Autodesk Inventor part; units mm, degrees
ref_plane "YZ Plane" through (0, 0, 0) normal (1, 0, 0) x (0, 1, 0)
ref_plane "XZ Plane" through (0, 0, 0) normal (0, 1, 0) x (-1, 0, 0)
ref_plane "XY Plane" through (0, 0, 0) normal (0, 0, 1) x (1, 0, 0)
sketch "Sketch1" plane through (0, 0, 0) normal (0, 1, 0) x (-1, 0, 0)
  line L0 (0, 0) -> (0, 19.05)
  line L1 (0, 19.05) -> (0.7937, 19.05)
  line L2 (0.7937, 19.05) -> (0.7938, 0.7937)
  line L3 (0.7938, 0.7937) -> (19.05, 0.7937)
  line L4 (19.05, 0.7937) -> (19.05, 0)
  line L5 (19.05, 0) -> (0, 0)
  dimension "d0" = 19.05
  dimension "d1" = 0.7937
extrude "Extrusion1" add sketch "Sketch1" along normal blind 76.2
sketch "Sketch2" plane through (0, 0, 19.05) normal (1, 0, 0) x (0, 0, -1)
  circle A0 centre (9.1281, 69.85) radius 3.3782
  circle A1 centre (9.1281, 44.45) radius 3.3782
  line L0 (0, 76.2) -> (19.05, 76.2)
  line L1 (0, 0) -> (0, 76.2)
  line L2 (18.2563, 0) -> (18.2563, 76.2)
  line L3 (18.2563, 38.1) -> (0, 38.1) construction
  line L4 (9.1281, 38.1) -> (9.1281, 76.2) construction
  dimension "d5" = 6.7564
  dimension "d18" = 25.4
  dimension "d19" = 6.35
extrude "Extrusion2" cut sketch "Sketch2" against normal through all
properties part number "Shooter Main Gear Guide Bar" material "Aluminum 6061"
Geometry check sheet. Reference: the model listing, model coordinates, mm. A direction names the side the tool comes from. Coordinates: 2 decimals unless noted, no trailing zeros. Write each loop counter-clockwise with the first axis right and the second up, starting at its lowest first coordinate (ties: lowest second). Pieces come first, ordered by that corner, then holes. Notation, with made-up numbers: M 73,-13.5 L 118,-13.5 A29 ccw 118,21.5 Z; hole C 70.25,-15.75 d5. An arc over 180 degrees is marked long. Use one line per item in the form item = value. Start each with the question number.
1) Set-up check for faces 1 (the flat face through (-0.3, 76.2, 5.3)), 2 (the flat face through (-10, 38, 0.794)): record each of +Z, -Z, +X, -X, +Y, -Y from which the full face is reachable in a straight line by a thin tool's end or side.
2) Release check for a two-part mould opening along Y. For faces 3 (the flat face through (-10, 38, 0)), 4 (the cylindrical face through (-0.391, 66.853, 8.363)), 5 (the flat face through (-0.3, 0, 5.3)), 6 (the cylindrical face through (-0.39, 41.15, 10.65)) record: pulls with the +Y half, pulls with the -Y half, needs draft (parallel to the pull), parting line crosses it, or undercut.
3) Section check C-C on y = 34. Enter the section's corners in (x, z).
4) Section check A-A on z = 10.25. Enter the section's corners in (x, y).
5) Section check B-B on y = 69.85. Enter the section's corners in (x, z), and give its area (3 significant figures).
6) Thickness scan on probe 1 along Z at (x, y) = (-0.2, 44.45); probe 2 along X at (y, z) = (71.5, 3); probe 3 along Z at (x, y) = (-7, 13). Record the ranges inside material, lowest first. Write a range as from..to.
7) Go/stop test with flat-tipped pins: pin 1 Ø4 at (x, y) = (-13.5, 61) entering from +Z; pin 2 Ø9 at (y, z) = (39.5, 6.5) entering from -X. Record where each tip stops, or that it passes through.
8) Section check D-D on x = -14.25. Enter the section's corners in (y, z), and give its area (3 significant figures).
Responses:
q1.face_1 = +Z, -Z, +X, -X, +Y
q1.face_2 = +Z, -X, +Y, -Y
q2.face_3 = needs draft
q2.face_4 = undercut
q2.face_5 = pulls with the -Y half
q2.face_6 = undercut
q3.outline = M -19.05,0 L 0,0 L 0,19.05 L -0.79,19.05 L -0.79,0.79 L -19.05,0.79 Z
q4.outline = M -0.79,0 L 0,0 L 0,41.09 L -0.79,41.09 Z; M -0.79,47.81 L 0,47.81 L 0,66.49 L -0.79,66.49 Z; M -0.79,73.21 L 0,73.21 L 0,76.2 L -0.79,76.2 Z
q5.outline = M -19.05,0 L 0,0 L 0,6.54 L -0.79,6.54 L -0.79,0.79 L -19.05,0.79 Z; M -0.79,13.3 L 0,13.3 L 0,19.05 L -0.79,19.05 Z
q5.area = 24.2 mm2
q6.probe_1 = 0..6.54, 13.3..19.05
q6.probe_2 = -0.79..0
q6.probe_3 = 0..0.79
q7.pin_1 = 0.79
q7.pin_2 = -0.79
q8.outline = M 0,0 L 76.2,0 L 76.2,0.79 L 0,0.79 Z
q8.area = 60.5 mm2
